from build123d import *

# Parameters (mm, degrees)
F0_W     = 30
F0_H     = 30
F0_W_2   = 26
F0_H_2   = 26
F1_DEPTH = 5
F0_W_3   = 39.9999991059
F0_H_3   = 39.9999991059
F2_DEPTH = 1
F3_W     = 2
F3_H     = 6
F3_W_2   = 26
F4_DEPTH = 2.2
F6_SIZE  = 0.99999


# Not quite as in the source:
# - a fillet or chamfer is up to 0.001 mm smaller than in the source, because OpenCascade refuses the exact size
# - a feature of the source that left no trace in its solid (it failed there, or was rolled back) is left out


with BuildPart() as f1:
    # F0 (on Top) → F1 (new body)
    with BuildSketch(Plane.XY):
        Rectangle(F0_W, F0_H)
        Rectangle(F0_W_2, F0_H_2, mode=Mode.SUBTRACT)
    extrude(amount=F1_DEPTH)

    # F0 (on Top) → F2 (join)
    with BuildSketch(Plane.XY):
        Rectangle(F0_W_3, F0_H_3)
        Rectangle(F0_W, F0_H, mode=Mode.SUBTRACT)
        Rectangle(F0_W_2, F0_H_2)
    extrude(amount=F2_DEPTH)

    # F3 (on face) → F4 (cut)
    with BuildSketch(Plane.XY.offset(5)):
        with Locations((-14, 0)):
            Rectangle(F3_W, F3_H)
        Rectangle(F3_W_2, F3_H)
        with Locations((14, 0)):
            Rectangle(F3_W, F3_H)
    extrude(amount=-F4_DEPTH, mode=Mode.SUBTRACT)

    # F6 (size 1 in the source; OpenCascade refuses exactly that, so slightly less here)
    f6_edges = [f1.edges().sort_by_distance(p)[0] for p in [
        (-20, 0, 0),
        (0, -20, 0),
        (20, 0, 0),
        (0, 20, 0),
    ]]
    chamfer(f6_edges, length=F6_SIZE)


solid = f1.part
CAD build for the part. Positions are in the model's coordinates, mm. A direction names the side the tool comes from. Round coordinates to 2 decimals unless told otherwise and drop trailing zeros. Order: outer loops, then holes, each group sorted by start corner. A loop starts at its lowest first (then second) coordinate and runs counter-clockwise, first axis right, second up. Notation, with made-up numbers: (52.25, 54) -> (80.25, 54) arc R32 ccw to (80.25, 93) -> close; hole circle Ø6 at (56, -1.5). An arc over 180 degrees is marked (long way). Write item = value, one per line. Start each with the question number.
(1) Which spindle directions (+Z, -Z, +X, -X, +Y, -Y) get a long thin tool onto all of the face, cutting with end or side? Do faces 1 (the flat face through (0, 15, 3)), 2 (the flat face through (-13, -0.2, 2.5)), 3 (the flat face through (14, 0, 2.8)). Say none if no direction does.
(2) Cut at A-A, the plane z = 3.4. List the corners of the cut face in (x, y), then the cut area to 3 significant figures.
(3) Pull direction X, two halves, no side cores. Call faces 4 (the flat face through (0, 0, 1)), 5 (the flat face through (15, -0.2, 2.5)), 6 (the flat face through (14, 3, 4)), 7 (the flat face through (0, 13, 3)): released by +X, released by -X, zero draft, split by the parting line, or undercut.
(4) Pin check, flat tips, straight feed: P1, Ø8, axis at x = 1.5, y = -1, coming from the +Z side; P2, Ø3, axis at y = 3.5, z = 4, coming from the -X side; P3, Ø2, axis at y = 1.5, z = 2.5, coming from the +X side. Stop position of each tip, or through.
(5) Probe line 1 (Y direction, x = -5, z = 3.45); line 2 (Y direction, x = -14, z = 4.6). List the from-to ranges inside material, lowest first. Write a range as [from, to].
Model answer:
q1.face_1 = +Z, +X, -X, +Y
q1.face_2 = +Z
q1.face_3 = +Z, +X, -X
q2.outline = (-15, -15) -> (15, -15) -> (15, -3) -> (13, -3) -> (13, -13) -> (-13, -13) -> (-13, -3) -> (-15, -3) -> close; (-15, 3) -> (-13, 3) -> (-13, 13) -> (13, 13) -> (13, 3) -> (15, 3) -> (15, 15) -> (-15, 15) -> close
q2.area = 200 mm2
q3.face_4 = undercut
q3.face_5 = released by +X
q3.face_6 = zero draft
q3.face_7 = undercut
q4.P1 = 1
q4.P2 = -15
q4.P3 = 15
q5.line_1 = [-15, -13], [13, 15]
q5.line_2 = [-15, -3], [3, 15]
